from build123d import *

# Parameters (mm, degrees)
SKETCH_1_R      = 21.5
EXTRUDE_1_DEPTH = 10


with BuildPart() as part:
    # Эскиз1 → Бобышка-Вытянуть1 (new body)
    with BuildSketch(Plane(origin=(0, 0, 0), x_dir=(1, 0, 0), z_dir=(0, 1, 0))):
        Polygon((0, 0), (120, 0), (120, 100), (40, 100), (40, 60), (0, 60), align=None)
        with Locations((77.5, 50)):
            Circle(SKETCH_1_R, mode=Mode.SUBTRACT)
    extrude(amount=EXTRUDE_1_DEPTH)


solid = part.part
Input: part model. Units: mm. Frame: model coordinates. A direction names the side the tool comes from. Round coordinates to 2 decimals unless told otherwise and drop trailing zeros. Loops run counter-clockwise (first coordinate to the right, second up) from the corner with the lowest first, then second, coordinate; pieces in that order, holes last. Notation, with made-up numbers: (57.25, 9) -> (89.25, 9) arc R13 cw to (89.25, 28) -> close; hole circle Ø4 at (-14, -20.5). An arc over 180 degrees is marked (long way). Answer as a JSON object with one key per item and string values. Group by question number.
1) Ray query, L1, parallel to Z at x = 77.5, y = 7.5; L2, parallel to X at y = 7, z = -50; L3, parallel to X at y = 7.75, z = -60.5. Return the intervals inside material, ascending.
2) Pin query (flat end, axial travel): pin 1 (5 mm diameter, centred on y = 7.5, z = -71, fed in from -X); pin 2 (3 mm diameter, centred on x = 26.5, y = 6.5, fed in from -Z). Return the tip coordinate at first contact, or that it passes through.
3) Draft query along X for faces 3 (the flat face through (0, 5, -30)), 4 (the cylindrical face through (98.007, 4.93, -56.458)), 5 (the flat face through (20, 5, -60)), 6 (the flat face through (120, 5, -49)). Return one class per face: +X half, -X half, draft (parallel to the pull), parting line (faces both ways), or undercut.
4) Reachability of faces 1 (the flat face through (81, 5, -100)), 2 (the flat face through (40, 5, -80)) from +Z, -Z, +X, -X, +Y, -Y: full face, straight path, thin tool, end or side. Return the list, or none.
5) Section query A-A on x = 77.5. Output: boundary loops of the cut face in (y, z).
6) Section query D-D on x = 22.5. Output: boundary loops of the cut face in (y, z), plus the area to 3 significant figures.
7) Section query C-C on y = 7.75. Output: boundary loops of the cut face in (x, z), plus the area to 3 significant figures.
8) Section query B-B on z = -50. Output: boundary loops of the cut face in (x, y).
Reply:
{
 "1": {"L1": "z = -100 to -71.5, -28.5 to 0", "L2": "x = 0 to 56, 99 to 120", "L3": "x = 40 to 58.74, 96.26 to 120"},
 "2": {"pin 1": "stops at x = 40", "pin 2": "stops at z = -60"},
 "3": {"face 3": "-X half", "face 4": "undercut", "face 5": "draft", "face 6": "+X half"},
 "4": {"face 1": "-Z, +X, -X, +Y, -Y", "face 2": "-Z, -X, +Y, -Y"},
 "5": {"outline": "(0, -100) -> (10, -100) -> (10, -71.5) -> (0, -71.5) -> close; (0, -28.5) -> (10, -28.5) -> (10, 0) -> (0, 0) -> close"},
 "6": {"outline": "(0, -60) -> (10, -60) -> (10, 0) -> (0, 0) -> close", "area": "600 mm2"},
 "7": {"outline": "(0, -60) -> (40, -60) -> (40, -100) -> (120, -100) -> (120, 0) -> (0, 0) -> close; hole circle Ø43 at (77.5, -50)", "area": "8,950 mm2"},
 "8": {"outline": "(0, 0) -> (56, 0) -> (56, 10) -> (0, 10) -> close; (99, 0) -> (120, 0) -> (120, 10) -> (99, 10) -> close"}
}
